```python
from build123d import *

# Parameters (mm, degrees)
SKETCH1_R           = 1.3
SKETCH1_R_2         = 1.2
BOSS_EXTRUDE1_DEPTH = 3


with BuildPart() as part:
    # Sketch1 → Boss-Extrude1 (new body)
    with BuildSketch(Plane(origin=(0, 0, 0), x_dir=(1, 0, 0), z_dir=(0, 1, 0))):
        Polygon((9.762662215, 65.669537047), (10.942509785, 65.669537047), (10.942509785, 84.984003028), (9.746724448, 84.984003028), (9.746724448, 93.703488322), (18.563219001, 93.703488322), (18.563219001, 84.984003028), (17.531387454, 84.984003028), (17.531387454, 65.669537047), (18.579156769, 65.669537047), (18.579156769, 63.040010061), (58.765583648, 63.040010061), (58.765583648, 65.796335383), (66.755517737, 65.796335383), (66.755517737, 85.084147443), (67.813967442, 85.084147443), (67.813967442, 93.803632737), (76.630461995, 93.803632737), (76.630461995, 85.084147443), (73.843318023, 85.084147443), (73.843318023, 57.076850089), (73.317218387, 57.076850089), (73.317218387, 7.739461046), (76.516310065, 7.739461046), (76.516310065, -0.980024248), (67.699815511, -0.980024248), (67.442656599, -1.105588805), (58.626162046, -1.105588805), (58.626162046, -0.977439081), (18.658261308, -0.977439081), (9.841766755, -0.977439081), (9.841766755, 7.742046212), (10.942509785, 7.742046212), (10.942509785, 56.950051753), (9.762662215, 56.950051753), align=None)
        with Locations(Location((14.154971724, 3.343745675, 0), (0, 0, 270))):
            Circle(SKETCH1_R, mode=Mode.SUBTRACT)
        with Locations(Location((63.154971724, 3.343745675, 0), (0, 0, 270))):
            Circle(SKETCH1_R, mode=Mode.SUBTRACT)
        with Locations(Location((14.154971724, 61.342146029, 0), (0, 0, 270))):
            Circle(SKETCH1_R, mode=Mode.SUBTRACT)
        with Locations(Location((63.154971698, 61.343745675, 0), (0, 0, 270))):
            Circle(SKETCH1_R, mode=Mode.SUBTRACT)
        with Locations(Location((72.154971724, 3.343745675, 0), (0, 0, 270))):
            Circle(SKETCH1_R_2, mode=Mode.SUBTRACT)
        with Locations(Location((72.154971724, 89.343745675, 0), (0, 0, 270))):
            Circle(SKETCH1_R_2, mode=Mode.SUBTRACT)
        with Locations(Location((14.154971724, 89.343745675, 0), (0, 0, 270))):
            Circle(SKETCH1_R_2, mode=Mode.SUBTRACT)
        Polygon((18.658261308, 7.742046212), (18.658261308, 6.082823098), (58.626162046, 6.082823098), (58.626162046, 7.613896488), (62.189336101, 7.739461046), (62.189336101, 57.076850089), (58.765583648, 57.076850089), (58.765583648, 58.793844452), (18.579156769, 58.793844452), (18.579156769, 56.950051753), (17.531387454, 56.950051753), (17.531387454, 7.742046212), align=None, mode=Mode.SUBTRACT)
    extrude(amount=BOSS_EXTRUDE1_DEPTH)


solid = part.part
```
Input: part model. Units: mm. Frame: model coordinates. A direction names the side the tool comes from. Round coordinates to 2 decimals unless told otherwise and drop trailing zeros. Loops run counter-clockwise (first coordinate to the right, second up) from the corner with the lowest first, then second, coordinate; pieces in that order, holes last. Notation, with made-up numbers: M -9.5,-24.75 L 7.5,-24.75 A14 cw 7.5,-12.75 Z; hole C -16,73.5 d2. An arc over 180 degrees is marked long. Answer in a Markdown table with one row per item. Add a question column.
1. Mould query, pull axis Z, two halves, no side actions, for faces 5 (the face through (63, 3, -43)), 6 (the face through (63, 1, -65.796)), 7 (the face through (14.21, 1.48, -62.64)). Classes: released by +Z, released by -Z, zero draft, split by the parting line, or undercut.
2. Ray query, probe 1 along Z at (x, y) = (63, 0.35); probe 2 along Z at (x, y) = (52, 1.55); probe 3 along X at (y, z) = (1, -76). Return the intervals inside material, ascending.
3. Section A-A (z = -70). Output: boundary loops of the cut face in (x, y).
4. Contact query for flat-ended pins moving along their axis: pin 1 (1 mm diameter, centred on y = 2.5, z = -63, fed in from -X); pin 2 (2 mm diameter, centred on x = 63.15, z = -3.34, fed in from +Y); pin 3 (3 mm diameter, centred on x = 31, z = -60.5, fed in from -Y); pin 4 (1.4 mm diameter, centred on x = 75, y = 1.5, fed in from +Z). Output: stop coordinate, or through.
5. Set-up query: faces 1 (the face through (10.943, 1, -32)), 2 (the face through (14, 1, -93.703)), 3 (the face through (73.843, 1, -71)), 4 (the face through (58.766, 1, -64)). Return all of +Z, -Z, +X, -X, +Y, -Y with unobstructed straight access to the full face (end or side cutting, diameter ignored); none if empty.
6. Section B-B (x = 56.5). Output: boundary loops of the cut face in (y, z), and give its area (3 significant figures).
7. Section C-C (y = 1.75). Give the number of separate pieces and of enclosed holes in the cut face, and give its area (3 significant figures).
Values follow:
| question | item | result |
|---|---|---|
| 1 | face 5 | zero draft |
| 1 | face 6 | released by -Z |
| 1 | face 7 | undercut |
| 2 | probe 1 | -65.8 to -62.63, -60.05 to -4.63, -2.05 to 1.11 |
| 2 | probe 2 | -63.04 to -58.79, -6.08 to 0.98 |
| 2 | probe 3 | 10.94 to 17.53, 66.76 to 73.84 |
| 3 | outline | M 10.94,0 L 17.53,0 L 17.53,3 L 10.94,3 Z; M 66.76,0 L 73.84,0 L 73.84,3 L 66.76,3 Z |
| 4 | pin 1 | x = 9.76 |
| 4 | pin 2 | through |
| 4 | pin 3 | y = 0 |
| 4 | pin 4 | z = 0.98 |
| 5 | face 1 | -X, +Y, -Y |
| 5 | face 2 | -Z, -X, +Y, -Y |
| 5 | face 3 | +X, +Y, -Y |
| 5 | face 4 | -Z, +Y, -Y |
| 6 | outline | M 0,-63.04 L 3,-63.04 L 3,-58.79 L 0,-58.79 Z; M 0,-6.08 L 3,-6.08 L 3,0.98 L 0,0.98 Z |
| 6 | area | 33.9 mm^2 |
| 7 | separate pieces | 1 |
| 7 | enclosed holes | 8 |
| 7 | area | 2,150 mm^2 |
